```python
from build123d import *

# Parameters (mm, degrees)
SKETCH_2_R          = 2.75
CUT_EXTRUDE_1_DEPTH = 27
SKETCH_3_R          = 2.75
CUT_EXTRUDE_2_DEPTH = 36.516660498
FILLET_1_R          = 0.5


with BuildPart() as part:
    # Sketch 1 → Revolve 1 (revolve)
    with BuildSketch(Plane(origin=(0, 0, 0), x_dir=(0, 0, -1), z_dir=(1, 0, 0))):
        with BuildLine():
            Line((17, 16.95), (22.5, 16.95))
            Line((22.5, 16.95), (22.5, 12.5))
            Line((22.5, 12.5), (-11.7, 12.5))
            Line((-11.7, 12.5), (-11.7, 16.95))
            Line((-11.7, 16.95), (0, 16.95))
            Line((0, 16.95), (0, 24.571324751))
            ThreePointArc((0, 24.571324751), (8.5, 26), (17, 24.571324751))
            Line((17, 24.571324751), (17, 16.95))
        make_face()
    revolve(axis=Axis((0, 0, 1108.809062344), (0, 0, -1)))

    # Sketch 2 → Cut-Extrude 1 (cut, through all)
    with BuildSketch(Plane(origin=(0, 0, 0), x_dir=(1, 0, 0), z_dir=(0, 1, 0))):
        with Locations((0, -5.85)):
            Circle(SKETCH_2_R)
    extrude(amount=CUT_EXTRUDE_1_DEPTH, mode=Mode.SUBTRACT)

    # Sketch 3 → Cut-Extrude 2 (cut, through all)
    with BuildSketch(Plane(origin=(0, 0, 0), x_dir=(0, 0, -1), z_dir=(0.866025404, 0.5, 0))):
        with Locations((-5.85, 0)):
            Circle(SKETCH_3_R)
    extrude(amount=-CUT_EXTRUDE_2_DEPTH, mode=Mode.SUBTRACT)

    # Fillet 1
    fillet_1_edges = [part.edges().sort_by_distance(p)[0] for p in [
        (0, -12.5, 11.7),
        (0, -12.5, -22.5),
        (0, -16.95, -22.5),
        (0, -16.95, 11.7),
    ]]
    fillet(fillet_1_edges, radius=FILLET_1_R)


solid = part.part
```
CAD build for the part. Positions are in the model's coordinates, mm. A direction names the side the tool comes from. Coordinates: 2 decimals unless noted, no trailing zeros. Loops run counter-clockwise (first coordinate to the right, second up) from the corner with the lowest first, then second, coordinate; pieces in that order, holes last. Notation, with made-up numbers: (0, 21) - (23, 21) arc R25 cw to (23, 33) - close; hole circle Ø3 at (12, -28). An arc over 180 degrees is marked (long way). Use CSV: the item, a comma, the result in double quotes. Start each with the question number.
Q1. Drop flat-ended pins along their axis: P1, Ø1.5, axis at x = 11.5, z = -17, coming from the -Y side; P2, Ø24.5, axis at x = -1, y = -11, coming from the -Z side; P3, Ø2, axis at y = 20, z = -12.5, coming from the -X side; P4, Ø5, axis at y = -13.5, z = 5.5, coming from the +X side. Give the stop position or say it passes through.
Q2. Cut at D-D, the plane z = 9.5. List the corners of the cut face in (x, y).
Q3. 3-axis set-ups, long thin cutter, end or side, ignore diameter. For faces 1 (the cylindrical face through (-0.358, 14.539, 3.123)), 2 (the flat face through (-5, -17, -17)), 3 (the flat face through (-5, 17, 0)): which of +Z, -Z, +X, -X, +Y, -Y reach the whole face in a straight line?
Q4. Cut at C-C, the plane z = 5.85. List the corners of the cut face in (x, y).
Q5. Probe probe 1 along Z at (x, y) = (0, 15.35); probe 2 along Z at (x, y) = (-14, 10); probe 3 along X at (y, z) = (-3.5, 9.5). List the from-to ranges inside material, lowest first. Write a range as from..to.
Q6. Cut at B-B, the plane y = 0. List the corners of the cut face in (x, z).
Q7. Cut at A-A, the plane x = 0. List the corners of the cut face in (y, z), then the cut area to 3 significant figures.
Q8. Two-plate mould, pull along X, no slides. Class faces 4 (the cylindrical face through (3.755, 11.923, -5.168)), 5 (the flat face through (-4.8, -12.3, -22.5)), 6 (the cylindrical face through (11.46, -12.49, 5.52)): +X half, -X half, draft (parallel to the pull), parting line (faces both ways), or undercut.
Here are the results:
1,P1,"y = -22.19"
1,P2,"z = -22.5"
1,P3,"x = -17.31"
1,P4,"x = 12.9"
2,outline,"circle Ø33.9 at (0, 0); hole circle Ø25 at (0, 0)"
3,face 1,"+Y"
3,face 2,"-Z"
3,face 3,"+Z"
4,outline,"(-15.86, -5.98) - (-11.94, -3.72) arc R12.5 cw to (-2.75, 12.19) - (-2.75, 16.73) arc R16.95 ccw to start; (-13.11, -10.74) arc R16.95 ccw (long way) to (2.75, 16.73) - (2.75, 12.19) arc R12.5 cw (long way) to (-9.19, -8.48) - close"
5,probe 1,"-22.5..3.1, 8.6..11.7"
5,probe 2,"-17..0"
5,probe 3,"-16.58..-12, 12..16.58"
6,outline,"(-24.57, -17) - (-16.95, -17) - (-16.95, -22) arc R0.5 ccw to (-16.45, -22.5) - (-13, -22.5) arc R0.5 ccw to (-12.5, -22) - (-12.5, 11.2) arc R0.5 ccw to (-13, 11.7) - (-16.45, 11.7) arc R0.5 ccw to (-16.95, 11.2) - (-16.95, 0) - (-24.57, 0) arc R26 ccw to start; (12.5, -22) arc R0.5 ccw to (13, -22.5) - (16.45, -22.5) arc R0.5 ccw to (16.95, -22) - (16.95, -17) - (24.57, -17) arc R26 ccw to (24.57, 0) - (16.95, 0) - (16.95, 11.2) arc R0.5 ccw to (16.45, 11.7) - (13, 11.7) arc R0.5 ccw to (12.5, 11.2) - close"
7,outline,"(-24.57, -17) - (-16.95, -17) - (-16.95, -22) arc R0.5 ccw to (-16.45, -22.5) - (-13, -22.5) arc R0.5 ccw to (-12.5, -22) - (-12.5, 11.2) arc R0.5 ccw to (-13, 11.7) - (-16.45, 11.7) arc R0.5 ccw to (-16.95, 11.2) - (-16.95, 0) - (-24.57, 0) arc R26 ccw to start; (12.5, -22) arc R0.5 ccw to (13, -22.5) - (16.45, -22.5) arc R0.5 ccw to (16.95, -22) - (16.95, -17) - (24.57, -17) arc R26 ccw to (24.57, 0) - (16.95, 0) - (16.95, 3.1) - (12.5, 3.1) - close; (12.5, 8.6) - (16.95, 8.6) - (16.95, 11.2) arc R0.5 ccw to (16.45, 11.7) - (13, 11.7) arc R0.5 ccw to (12.5, 11.2) - close"
7,area,"571 mm2"
8,face 4,"undercut"
8,face 5,"draft"
8,face 6,"parting line"
